Here's how the part is built. I have some questions about the finished solid (model axes, mm). A direction names the side the tool comes from. Round coordinates to 2 decimals unless told otherwise and drop trailing zeros. Loops run counter-clockwise (first coordinate to the right, second up) from the corner with the lowest first, then second, coordinate; pieces in that order, holes last. Notation, with made-up numbers: (39.25, -39.5) -> (59.25, -39.5) arc R19 ccw to (59.25, -23.5) -> close; hole circle Ø2 at (77, 80). An arc over 180 degrees is marked (long way). Use CSV: the item, a comma, the result in double quotes. Start each with the question number.
from build123d import *

# Parameters (mm, degrees)
F0_R     = 5
F0_R_2   = 4
F1_DEPTH = 8.5


with BuildPart() as f1:
    # F0 (on Top) → F1 (new body, symmetric)
    with BuildSketch(Plane.XY):
        with BuildLine():
            Line((15.090626, 16.689009), (-21.443711, 49.724285))
            ThreePointArc((-21.443711, 49.724285), (-49.611346, 49.382679), (-49.497475, 21.213203))
            Line((-49.497475, 21.213203), (-45.750738, 18.269213))
            Line((-45.750738, 18.269213), (-22.5, 0))
            Line((-22.5, 0), (-22.5, -26.8))
            ThreePointArc((-22.5, -26.8), (0, -49.3), (22.5, -26.8))
            Line((22.5, -26.8), (22.5, 0))
            ThreePointArc((22.5, 0), (20.5644, 9.129921), (15.090626, 16.689009))
        make_face()
        with Locations((0, -26.8)):
            Circle(F0_R, mode=Mode.SUBTRACT)
        Circle(F0_R_2, mode=Mode.SUBTRACT)
        with Locations((-35.355339, 35.355339)):
            Circle(F0_R_2, mode=Mode.SUBTRACT)
    extrude(amount=F1_DEPTH, both=True)


solid = f1.part
Q1. If we mould it in two halves opening along X, with no side actions, what happens to faces 1 (the flat face through (-2.921, 32.975, 0.119)), 2 (the cylindrical face through (-0.495, -49.295, 0.119)), 3 (the cylindrical face through (-31.54, 36.56, -0.12))? For each: pulls with the +X half, pulls with the -X half, needs draft (parallel to the pull), parting line crosses it, or undercut.
Q2. Will these pins go through, and if not, where does the flat tip stop? pin 1 Ø13 at (x, y) = (0, -26.8) entering from +Z; pin 2 Ø10 at (x, z) = (-17.5, 6.5) entering from -Y; pin 3 Ø8.5 at (y, z) = (-16.5, 2) entering from -X; pin 4 Ø8 at (x, z) = (1, -4.5) entering from +Y.
Q3. I want a section at B-B, the plane x = 0. List the corners of the cut face in (y, z) for me, then the cut area to 3 significant figures.
Q4. I want a section at A-A, the plane z = -6. List the corners of the cut face in (x, y) for me.
Q5. I want a section at C-C, the plane y = -14.5. List the corners of the cut face in (x, z) for me, then the cut area to 3 significant figures.
Q6. For faces 4 (the flat face through (-22.5, -13, 0)), 5 (the cylindrical face through (-0.867, -3.905, -0.119)), which set-ups out of +Z, -Z, +X, -X, +Y, -Y let a thin tool reach every point of the face, with its end or its side?
Q7. I want a section at D-D, the plane x = -41. List the corners of the cut face in (y, z) for me.
Q8. I need wall thicknesses on line 1 along Y through (x, z) = (0, -3.5); line 2 along X through (y, z) = (-9, 7.5); line 3 along X through (y, z) = (-23, 7.5). Which ranges of each line are inside material? Lowest first, please.
Values found:
1,face 1,"pulls with the +X half"
1,face 2,"parting line crosses it"
1,face 3,"undercut"
2,pin 1,"z = 8.5"
2,pin 2,"y = -45.51"
2,pin 3,"x = -22.5"
2,pin 4,"y = 33.05"
3,outline,"(-49.3, -8.5) -> (-31.8, -8.5) -> (-31.8, 8.5) -> (-49.3, 8.5) -> close; (-21.8, -8.5) -> (-4, -8.5) -> (-4, 8.5) -> (-21.8, 8.5) -> close; (4, -8.5) -> (30.33, -8.5) -> (30.33, 8.5) -> (4, 8.5) -> close"
3,area,"1,050 mm2"
4,outline,"(-49.5, 21.21) -> (-22.5, 0) -> (-22.5, -26.8) arc R22.5 ccw to (22.5, -26.8) -> (22.5, 0) arc R22.5 ccw to (15.09, 16.69) -> (-21.44, 49.72) arc R20 ccw to start; hole circle Ø8 at (-35.36, 35.36); hole circle Ø10 at (0, -26.8); hole circle Ø8 at (0, 0)"
5,outline,"(-22.5, -8.5) -> (22.5, -8.5) -> (22.5, 8.5) -> (-22.5, 8.5) -> close"
5,area,"765 mm2"
6,face 4,"+Z, -Z, -X, -Y"
6,face 5,"+Z, -Z"
7,outline,"(14.54, -8.5) -> (54.54, -8.5) -> (54.54, 8.5) -> (14.54, 8.5) -> close"
8,line 1,"-49.3 to -31.8, -21.8 to -4, 4 to 30.33"
8,line 2,"-22.5 to 22.5"
8,line 3,"-22.5 to -3.25, 3.25 to 22.5"
